Geometry check sheet. Reference: the model listing, model coordinates, mm. A direction names the side the tool comes from. Round coordinates to 2 decimals unless told otherwise and drop trailing zeros. Write each loop counter-clockwise with the first axis right and the second up, starting at its lowest first coordinate (ties: lowest second). Pieces come first, ordered by that corner, then holes. Notation, with made-up numbers: M -21.75,2.5 L 27.25,2.5 A9 ccw 27.25,15.5 Z; hole C 17.25,42.25 d4. An arc over 180 degrees is marked long. Put each result on its own line as item: value. Start each with the question number.
(1) Tool access check on faces 5 (the flat face through (21, 10, -6.5)), 6 (the flat face through (34, 17, -12)), 7 (the cylindrical face through (20.474, 16.339, -3.965)), 8 (the flat face through (21, 10, -1.5)). Record the directions out of +Z, -Z, +X, -X, +Y, -Y that give a thin tool (end or side, any length) a straight path to the whole face; none if there is none.
(2) Gauge pin test, flat ends, axial feed: pin 1 (10 mm diameter, centred on x = 7.5, y = 9, fed in from +Z); pin 2 (4 mm diameter, centred on y = 7, z = -3, fed in from -X); pin 3 (5.5 mm diameter, centred on x = 20, y = 11.5, fed in from -Z); pin 4 (20 mm diameter, centred on x = 10.5, z = -13, fed in from -Y). Record the tip position at first contact, or that the pin passes through.
(3) Material ranges on probe 1 along X at (y, z) = (2.7, 22.5); probe 2 along Y at (x, z) = (-1, -25.5); probe 3 along X at (y, z) = (9.75, -4), recorded low to high.
(4) Section check B-B on x = 20.65. Record the cut outline in (y, z).
(5) Section check A-A on y = 15. Record the cut outline in (x, z).
(6) Section check C-C on z = -47.5. Record the cut outline in (x, y), then the cut area to 3 significant figures.
(7) Section check D-D on x = -19. Record the cut outline in (y, z), then the cut area to 3 significant figures.
(8) Mould release check, pull along Z, two halves, no side actions. Record for faces 1 (the flat face through (11, 21, 12.5)), 2 (the cylindrical face through (28.35, 2.46, 24.07)), 3 (the flat face through (13, 2, -52.5)), 4 (the flat face through (49, 2, -12)): pulls with the +Z half, pulls with the -Z half, needs draft (parallel to the pull), parting line crosses it, or undercut.
from build123d import *

# Parameters (mm, degrees)
SKETCH_1_R          = 1.7
EXTRUDE_1_DEPTH     = 5
EXTRUDE_2_DEPTH     = 15
SKETCH_3_W          = 58
SKETCH_3_H          = 50
EXTRUDE_3_DEPTH     = 5
SKETCH_4_W          = 5
SKETCH_4_H          = 20
EXTRUDE_4_DEPTH     = 7
SKETCH_6_R          = 1.35
CUT_EXTRUDE_1_DEPTH = 8
FILLET_1_R          = 5


with BuildPart() as part:
    # 草图1 → 凸台-拉伸1 (new body)
    with BuildSketch(Plane(origin=(0, 0, 0), x_dir=(1, 0, 0), z_dir=(0, 1, 0))):
        Polygon((24, 27.5), (24, -27.5), (49, -27.5), (49, 52.5), (-24, 52.5), (-24, 27.5), align=None)
        with Locations(Location((29, -22.5, 0), (0, 0, 270))):
            Circle(SKETCH_1_R, mode=Mode.SUBTRACT)
        with Locations(Location((44, 47.5, 0), (0, 0, 270))):
            Circle(SKETCH_1_R, mode=Mode.SUBTRACT)
        with Locations(Location((-19, 47.5, 0), (0, 0, 270))):
            Circle(SKETCH_1_R, mode=Mode.SUBTRACT)
    extrude(amount=EXTRUDE_1_DEPTH)

    # 草图2 → 凸台-拉伸2 (add)
    with BuildSketch(Plane(origin=(0, 5, 0), x_dir=(1, 0, 0), z_dir=(0, 1, 0))):
        Polygon((-24, 37.5), (-24, 27.5), (24, 27.5), (24, -12.5), (34, -12.5), (34, 37.5), align=None)
    extrude(amount=EXTRUDE_2_DEPTH)

    # 草图3 → 凸台-拉伸3 (add)
    with BuildSketch(Plane(origin=(0, 20, 0), x_dir=(1, 0, 0), z_dir=(0, 1, 0))):
        with Locations((5, 12.5)):
            Rectangle(SKETCH_3_W, SKETCH_3_H)
    extrude(amount=EXTRUDE_3_DEPTH)

    # 草图4 → 凸台-拉伸4 (add)
    with BuildSketch(Plane.ZY.offset(-24)):
        with Locations((-4, 10)):
            Rectangle(SKETCH_4_W, SKETCH_4_H)
    extrude(amount=EXTRUDE_4_DEPTH)

    # 草图6 → 切除-拉伸1 (cut)
    with BuildSketch(Plane.XY.offset(-1.5)):
        with Locations((20.65, 15)):
            Circle(SKETCH_6_R)
        with Locations((20.65, 5)):
            Circle(SKETCH_6_R)
    extrude(amount=-CUT_EXTRUDE_1_DEPTH, mode=Mode.SUBTRACT)

    # 圆角1
    fillet_1_edges = [part.edges().sort_by_distance(p)[0] for p in [
        (34, 5, -12.5),
        (5, 5, -37.5),
        (29, 5, 12.5),
    ]]
    fillet(fillet_1_edges, radius=FILLET_1_R)


solid = part.part
Answers follow:
1. face 5: -X, -Y
1. face 6: +Z, -Z, +X, +Y
1. face 7: +Z
1. face 8: +Z, -X, -Y
2. pin 1: stops at z = -27.5
2. pin 2: stops at x = 17
2. pin 3: stops at z = -37.66
2. pin 4: stops at y = 0
3. probe 1: x = 24 to 27.3, 30.7 to 49
3. probe 2: y = 20 to 25
3. probe 3: x = 17 to 34.01
4. outline: M 0,-52.5 L 5,-52.5 L 5,-42.5 A5 cw 10,-37.5 L 25,-37.5 L 25,12.5 L 20,12.5 L 20,-1.5 L 16.35,-1.5 L 16.35,-6.5 L 20,-6.5 L 20,-27.5 L 0,-27.5 Z; M 0,-6.5 L 3.65,-6.5 L 3.65,-1.5 L 0,-1.5 Z; M 6.35,-6.5 L 13.65,-6.5 L 13.65,-1.5 L 6.35,-1.5 Z
5. outline: M -24,-37.5 L 34,-37.5 L 34,12.5 L 24,12.5 L 24,-1.5 L 22,-1.5 L 22,-6.5 L 24,-6.5 L 24,-27.5 L -24,-27.5 Z; M 17,-6.5 L 19.3,-6.5 L 19.3,-1.5 L 17,-1.5 Z
6. outline: M -24,0 L -20.7,0 L -20.7,5 L -24,5 Z; M -17.3,0 L 42.3,0 L 42.3,5 L -17.3,5 Z; M 45.7,0 L 49,0 L 49,5 L 45.7,5 Z
6. area: 331 mm^2
7. outline: M 0,-52.5 L 5,-52.5 L 5,-49.2 L 0,-49.2 Z; M 0,-45.8 L 5,-45.8 L 5,-42.5 A5 cw 10,-37.5 L 25,-37.5 L 25,12.5 L 20,12.5 L 20,-27.5 L 0,-27.5 Z
7. area: 513 mm^2
8. face 1: pulls with the +Z half
8. face 2: undercut
8. face 3: pulls with the -Z half
8. face 4: needs draft
